Autodesk Inventor part; units mm, degrees
ref_plane "YZ Plane" through (0, 0, 0) normal (1, 0, 0) x (0, 1, 0)
ref_plane "XZ Plane" through (0, 0, 0) normal (0, 1, 0) x (-1, 0, 0)
ref_plane "XY Plane" through (0, 0, 0) normal (0, 0, 1) x (1, 0, 0)
sketch "スケッチ1" plane through (0, 0, 0) normal (0, 0, 1) x (1, 0, 0)
  circle A0 centre (0, 0) radius 2.25
  circle A1 centre (0, 0) radius 1.3
  dimension "d0" = 4.5
  dimension "d6" = 2.6
extrude "押し出し1" add sketch "スケッチ1" along normal blind 2.5 contours A0 | A1
sketch "スケッチ2" plane through (0, 0, 2.5) normal (0, 0, 1) x (1, 0, 0)
  circle A0 centre (0, 0) radius 2.25
  line L0 (-0.3947, -1.0851) -> (-1.1371, -0.2007)
  line L1 (-1.1371, -0.2007) -> (-0.7424, 0.8844)
  line L2 (-0.7424, 0.8844) -> (0.3947, 1.0851)
  line L3 (0.3947, 1.0851) -> (1.1371, 0.2007)
  line L4 (1.1371, 0.2007) -> (0.7424, -0.8844)
  line L5 (0.7424, -0.8844) -> (-0.3947, -1.0851)
  dimension "d3" = 2
extrude "押し出し2" cut sketch "スケッチ2" against normal blind 1.1 contours L0 L1 L2 L3 L4 L5
extrude "押し出し3" add sketch "スケッチ1" against normal blind 6 contours A1
thread "ねじ1"
properties part number "ネジキャップM2.6L6ステンレス" material "ステンレス鋼"
Model file for the job. Use its own axes, mm. A direction names the side the tool comes from. Give positions to 0.01 mm unless a question says otherwise; leave off trailing zeros. Write each loop counter-clockwise with the first axis right and the second up, starting at its lowest first coordinate (ties: lowest second). Pieces come first, ordered by that corner, then holes. Notation, with made-up numbers: (52, 38.5) - (57, 38.5) arc R14 cw to (57, 57.5) - close; hole circle Ø2 at (66, 1.5). An arc over 180 degrees is marked (long way). One line per question, with ' | ' between items. Start each with the question number.
(1) Pin check, flat tips, straight feed: P1, Ø2, axis at x = 1.5, z = 1.5, coming from the -Y side; P2, Ø1.7, axis at x = 0.5, y = 0.5, coming from the +Z side; P3, Ø2, axis at x = 1.5, z = 1.5, coming from the +Y side; P4, Ø1.5, axis at x = 1, z = -1.5, coming from the -Y side. Stop position of each tip, or through.
(2) Slice it at D-D on y = 0. Write the cut outline in (x, z), plus the area to 3 significant figures.
(3) 3-axis set-ups, long thin cutter, end or side, ignore diameter. For faces 1 (the face through (0, -1.5, 0)), 2 (the face through (-0.8, -0.6, 2)), 3 (the face through (1, 1, 2.5)): which of +Z, -Z, +X, -X, +Y, -Y reach the whole face in a straight line?
(4) Slice it at C-C on z = 1. Write the cut outline in (x, y).
(5) Two-plate mould, pull along Y, no slides. Class faces 4 (the face through (-0.29, -2.23, 1.23)), 5 (the face through (-0.182, 0.983, 1.958)), 6 (the face through (0, 0, -6)): +Y half, -Y half, draft (parallel to the pull), parting line (faces both ways), or undercut.
(6) Slice it at B-B on y = -1.2. Write the cut outline in (x, z).
(7) Wall check: line 1 along Z through (x, y) = (1.8, -1.2); line 2 along Z through (x, y) = (0.6, 0.6); line 3 along X through (y, z) = (-0.75, -2.5). Give the ranges that are in metal, low to high. Write a range as from..to.
(8) Slice it at A-A on x = 0.3. Write the cut outline in (y, z), plus the area to 3 significant figures.
Results below:
1) P1: y = -2.19 | P2: z = 2.5 | P3: y = 2.19 | P4: y = -1.28
2) outline: (-2.25, 0) - (-1.3, 0) - (-1.3, -6) - (1.3, -6) - (1.3, 0) - (2.25, 0) - (2.25, 2.5) - (1.06, 2.5) - (1.06, 1.4) - (-1.06, 1.4) - (-1.06, 2.5) - (-2.25, 2.5) - close | area: 24.5 mm^2
3) face 1: -Z | face 2: +Z | face 3: +Z, +X, -X, +Y, -Y
4) outline: circle Ø4.5 at (0, 0)
5) face 4: parting line | face 5: undercut | face 6: draft
6) outline: (-1.9, 0) - (-0.5, 0) - (-0.5, -6) - (0.5, -6) - (0.5, 0) - (1.9, 0) - (1.9, 2.5) - (-1.9, 2.5) - close
7) line 1: 0..2.5 | line 2: -6..1.4 | line 3: -1.06..1.06
8) outline: (-2.23, 0) - (-1.26, 0) - (-1.26, -6) - (1.26, -6) - (1.26, 0) - (2.23, 0) - (2.23, 2.5) - (1.07, 2.5) - (1.07, 1.4) - (-0.96, 1.4) - (-0.96, 2.5) - (-2.23, 2.5) - close | area: 24.1 mm^2
